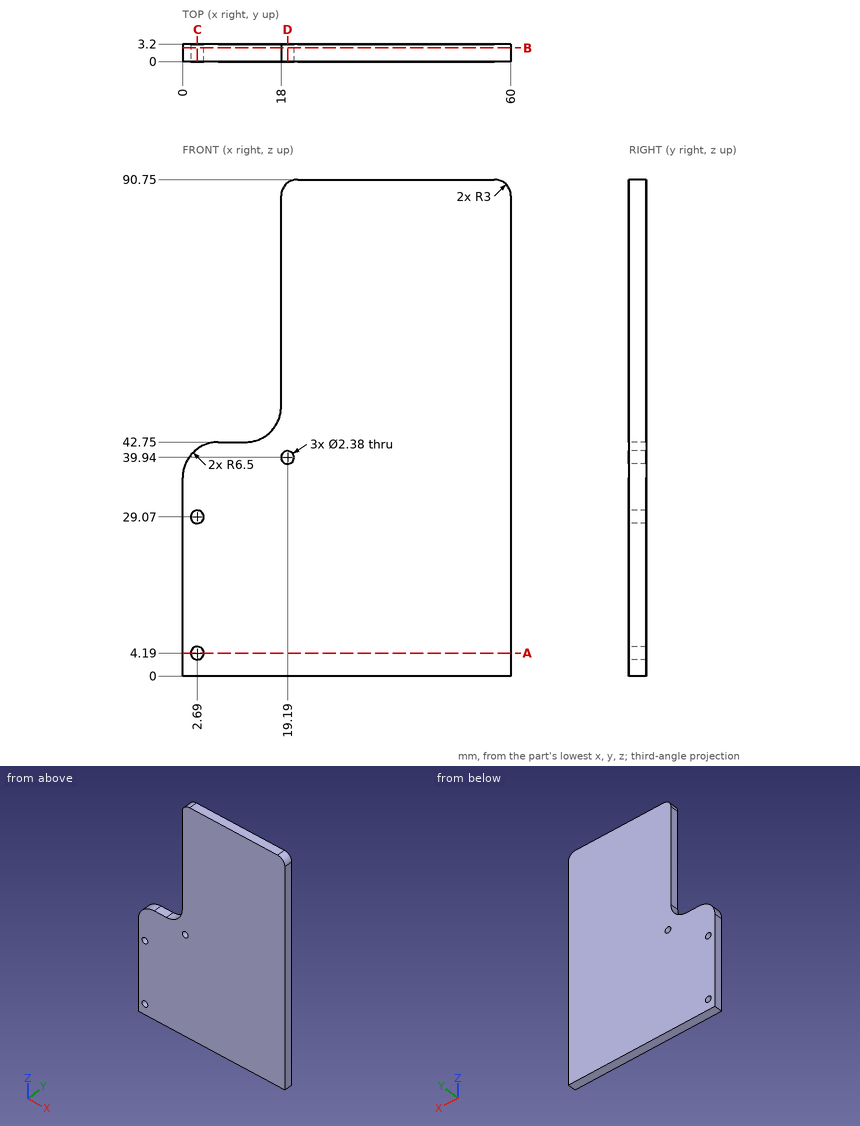
Geometry: see drawing. Coordinates: mm, zero at the bounding-box minimum. Coordinates: 2 decimals unless noted, no trailing zeros. Loops run counter-clockwise (first coordinate to the right, second up) from the corner with the lowest first, then second, coordinate; pieces in that order, holes last. Notation, with made-up numbers: (12, 32) - (54, 32) arc R15 ccw to (54, 49) - close; hole circle Ø5 at (67, 37.5). An arc over 180 degrees is marked (long way). Answer in a Markdown table with one row per item.
(1) Cut plane D-D on x = 19.19. Output: boundary loops of the cut face in (y, z), plus the area to 3 significant figures.
Model answer:
| item | result |
|---|---|
| outline | (0, 0) - (3.2, 0) - (3.2, 38.75) - (0, 38.75) - close; (0, 41.13) - (3.2, 41.13) - (3.2, 90.14) - (0, 90.14) - close |
| area | 281 mm² |
(2) Material intervals for L1, parallel to Z at x = 2.69, y = 1.05; L2, parallel to Z at x = 9.5, y = 1.5; L3, parallel to X at y = 1.2, z = 64.5, sorted ascending. Write a range as from..to.
Model answer:
| item | result |
|---|---|
| L1 | z = 0..3, 5.38..27.88, 30.26..41.52 |
| L2 | z = 0..42.75 |
| L3 | x = 18..60 |
(3) Cut plane A-A on z = 4.19. Output: boundary loops of the cut face in (x, y).
Model answer:
| item | result |
|---|---|
| outline | (0, 0) - (1.5, 0) - (1.5, 3.2) - (0, 3.2) - close; (3.88, 0) - (60, 0) - (60, 3.2) - (3.88, 3.2) - close |
(4) Pin query (flat end, axial travel): P1, Ø1, axis at x = 9, y = 1.5, coming from the +Z side; P2, Ø1.6, axis at y = 1, z = 77, coming from the -X side; P3, Ø1.4, axis at x = 2.69, z = 4.19, coming from the +Y side. Return the tip coordinate at first contact, or that it passes through.
Model answer:
| item | result |
|---|---|
| P1 | stops at z = 42.75 |
| P2 | stops at x = 18 |
| P3 | passes through |
(5) Cut plane C-C on x = 2.69. Output: boundary loops of the cut face in (y, z), plus the area to 3 significant figures.
Model answer:
| item | result |
|---|---|
| outline | (0, 0) - (3.2, 0) - (3.2, 3) - (0, 3) - close; (0, 5.38) - (3.2, 5.38) - (3.2, 27.88) - (0, 27.88) - close; (0, 30.26) - (3.2, 30.26) - (3.2, 41.52) - (0, 41.52) - close |
| area | 118 mm² |
(6) Cut plane B-B on y = 2.5. Output: boundary loops of the cut face in (x, z).
Model answer:
| item | result |
|---|---|
| outline | (0, 0) - (60, 0) - (60, 87.75) arc R3 ccw to (57, 90.75) - (21, 90.75) arc R3 ccw to (18, 87.75) - (18, 49.25) arc R6.5 cw to (11.5, 42.75) - (6.5, 42.75) arc R6.5 ccw to (0, 36.25) - close; hole circle Ø2.38 at (2.69, 4.19); hole circle Ø2.38 at (2.69, 29.07); hole circle Ø2.38 at (19.19, 39.94) |
